The model under review builds one solid part; all positions refer to its coordinate system, in mm. Coordinates: 2 decimals unless noted, no trailing zeros. Write each loop counter-clockwise with the first axis right and the second up, starting at its lowest first coordinate (ties: lowest second). Pieces come first, ordered by that corner, then holes. Notation, with made-up numbers: (30.25, -10.5) -> (70.25, -10.5) arc R29 ccw to (70.25, 25.5) -> close; hole circle Ø3 at (55.25, 44). An arc over 180 degrees is marked (long way). Write each question's results on one line, items separated by ' | '.
```python
from build123d import *

# Parameters (mm, degrees)
EXTRUDE_1_DEPTH        = 10
FILLET_1_R             = 6
HOLE_WIZARD_M8_1_D     = 6.8
HOLE_WIZARD_M8_1_DEPTH = 19.75
HOLE_WIZARD_M8_1_TIP   = 2.042926105
FILLET_2_R             = 50


with BuildPart() as part:
    # 草图1 → 凸台-拉伸1 (new body)
    with BuildSketch(Plane.XY):
        with BuildLine():
            Line((-350, 0), (350, 0))
            Line((350, 0), (410, -40))
            Line((410, -40), (680, -40))
            Line((680, -40), (680, -98))
            Line((680, -98), (429.970360472, -98))
            Line((429.970360472, -98), (330, -168))
            Line((330, -168), (310, -168))
            Line((310, -168), (310, -98))
            Line((310, -98), (225, -98))
            Line((225, -98), (225, -88))
            Line((225, -88), (244.858994383, -74.458569423))
            ThreePointArc((244.858994383, -74.458569423), (251.722364739, -54.841267835), (235, -42.5))
            Line((235, -42.5), (-235, -42.5))
            ThreePointArc((-235, -42.5), (-251.722364739, -54.841267835), (-244.858994383, -74.458569423))
            Line((-244.858994383, -74.458569423), (-225, -88))
            Line((-225, -88), (-225, -98))
            Line((-225, -98), (-310, -98))
            Line((-310, -98), (-310, -168))
            Line((-310, -168), (-330, -168))
            Line((-330, -168), (-429.970360472, -98))
            Line((-429.970360472, -98), (-680, -98))
            Line((-680, -98), (-680, -40))
            Line((-680, -40), (-410, -40))
            Line((-410, -40), (-350, 0))
        make_face()
    extrude(amount=EXTRUDE_1_DEPTH)

    # 圆角1
    fillet_1_edges = [part.edges().sort_by_distance(p)[0] for p in [
        (-350, 0, 5),
        (350, 0, 5),
        (410, -40, 5),
        (-410, -40, 5),
    ]]
    fillet(fillet_1_edges, radius=FILLET_1_R)

    # M8 螺纹孔1
    with Locations(Plane.XY.offset(10)):
        with Locations((0, -27.5)):
            Hole(HOLE_WIZARD_M8_1_D / 2, depth=HOLE_WIZARD_M8_1_DEPTH)
            with Locations((0, 0, -(HOLE_WIZARD_M8_1_DEPTH + HOLE_WIZARD_M8_1_TIP / 2))):  # 118° drill point
                Cone(0, HOLE_WIZARD_M8_1_D / 2, HOLE_WIZARD_M8_1_TIP, mode=Mode.SUBTRACT)

    # 圆角2
    fillet_2_edges = [part.edges().sort_by_distance(p)[0] for p in [
        (429.970360472, -98, 5),
        (-429.970360472, -98, 5),
    ]]
    fillet(fillet_2_edges, radius=FILLET_2_R)


solid = part.part
```
Q1. For line 1 (Y direction, x = 0, z = 4.5); line 2 (Y direction, x = -575.5, z = 6); line 3 (Y direction, x = 148, z = 5), list the stretches that pass through material, from the lowest coordinate up. Write a range as from..to.
Solution:
line 1: -42.5..-30.9, -24.1..0 | line 2: -98..-40 | line 3: -42.5..0
Q2. Clearance check with flat-ended pins moving along their axes: P1, Ø6, axis at y = -109, z = 2.5, coming from the -X side; P2, Ø3, axis at x = 271.5, z = 4.5, coming from the -Y side; P3, Ø3, axis at x = 12.5, z = 6, coming from the -Y side. State where each tip first meets the part, or that it passes through.
Solution:
P1: x = -418.61 | P2: y = -98 | P3: y = -42.5
Q3. Add section B-B (y = -122). Write out the cut boundary in (x, z), plus the area to 3 significant figures.
Solution:
outline: (-395.69, 0) -> (-310, 0) -> (-310, 10) -> (-395.69, 10) -> close; (310, 0) -> (395.69, 0) -> (395.69, 10) -> (310, 10) -> close | area: 1,710 mm²
Q4. Add section C-C (x = 572.5). Write out the cut boundary in (y, z).
Solution:
outline: (-98, 0) -> (-40, 0) -> (-40, 10) -> (-98, 10) -> close
Q5. Add section D-D (x = 273). Write out the cut boundary in (y, z).
Solution:
outline: (-98, 0) -> (0, 0) -> (0, 10) -> (-98, 10) -> close
